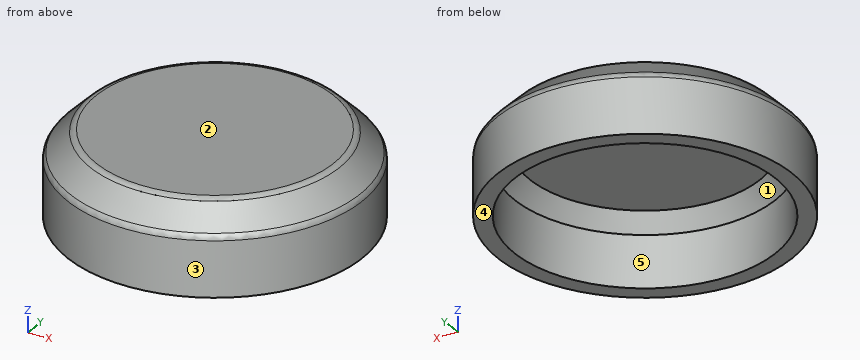
```python
from build123d import *

# Parameters (mm, degrees)
F0_R     = 17.5
F1_DEPTH = 10
F2_SIZE  = 3
F3_R     = 1
F4_T     = -2


with BuildPart() as f1:
    # F0 (on Top) → F1 (new body)
    with BuildSketch(Plane.XY):
        Circle(F0_R)
    extrude(amount=F1_DEPTH)

    # F2
    f2_edges = [f1.edges().sort_by_distance(p)[0] for p in [
        (-17.5, 0, 10),
    ]]
    chamfer(f2_edges, length=F2_SIZE)

    # F3
    f3_edges = [f1.edges().sort_by_distance(p)[0] for p in [
        (16, 0, 8.5),
        (-17.5, 0, 7),
        (-14.5, 0, 10),
    ]]
    fillet(f3_edges, radius=F3_R)

    # F4
    f4_openings = [f1.faces().sort_by_distance(p)[0] for p in [
        (0, 0, 0),
    ]]
    offset(amount=F4_T, openings=f4_openings)


solid = f1.part
```
CAD build for the part. Positions are in the model's coordinates, mm. Face numbers are marked on the shaded views. A direction names the side the tool comes from. Round coordinates to 2 decimals unless told otherwise and drop trailing zeros. Write each loop counter-clockwise with the first axis right and the second up, starting at its lowest first coordinate (ties: lowest second). Pieces come first, ordered by that corner, then holes. Notation, with made-up numbers: (2.5, -2) - (47.5, -2) arc R25 cw to (47.5, 21) - close; hole circle Ø2 at (36.25, -32). An arc over 180 degrees is marked (long way). Return JSON: item names as keys, results as strings. Group by question number.
Item 1: Band-saw the part on A-A on z = 4.5. List the corners of the cut face in (x, y), plus the area to 3 significant figures.
Item 2: Probe probe 1 along X at (y, z) = (0, 2.5); probe 2 along Z at (x, y) = (-8.5, 2). List the from-to ranges inside material, lowest first.
Item 3: 3-axis set-ups, long thin cutter, end or side, ignore diameter. For the marked faces 4 and 5: which of +Z, -Z, +X, -X, +Y, -Y reach the whole face in a straight line?
Item 4: Mould opens along X. For the marked faces 1, 2 and 3 say: +X half, -X half, draft (parallel to the pull), parting line (faces both ways), or undercut.
Item 5: Flat gauge pins, fed straight in: pin 1 Ø2 at (x, z) = (-6.5, 7) entering from +Y; pin 2 Ø5 at (x, z) = (8, 7) entering from -Y; pin 3 Ø1.5 at (x, z) = (-5.5, 8) entering from -Y. Where does each tip first touch, or does it go through?
Resolved:
{
 "1": {"outline": "circle Ø35 at (0, 0); hole circle Ø31 at (0, 0)", "area": "207 mm²"},
 "2": {"probe 1": "x = -17.5 to -15.5, 15.5 to 17.5", "probe 2": "z = 8 to 10"},
 "3": {"face 4": "-Z, +X, -X, +Y, -Y", "face 5": "-Z"},
 "4": {"face 1": "undercut", "face 2": "draft", "face 3": "parting line"},
 "5": {"pin 1": "stops at y = 16.59", "pin 2": "stops at y = -16.6", "pin 3": "stops at y = -16.39"}
}
